from build123d import *

# Parameters (mm, degrees)
SALIENTE_EXTRUIR1_DEPTH = 0.8
SALIENTE_EXTRUIR2_DEPTH = 8
CROQUIS3_R              = 2.25
CORTAR_EXTRUIR1_DEPTH   = 0.8


with BuildPart() as part:
    # Croquis1 → Saliente-Extruir1 (new body)
    with BuildSketch(Plane.XY):
        with BuildLine():
            Line((-68.221491284, 9.846072283), (-68.221491284, 13.429873796))
            Line((-68.221491284, 13.429873796), (-62.221491284, 13.429873796))
            Line((-62.221491284, 13.429873796), (-62.221491284, 9.846072283))
            ThreePointArc((-62.221491284, 9.846072283), (-59.564637034, 8.086728046), (-57.805292797, 5.429873796))
            Line((-57.805292797, 5.429873796), (-54.221491284, 5.429873796))
            Line((-54.221491284, 5.429873796), (-54.221491284, -0.570126204))
            Line((-54.221491284, -0.570126204), (-57.805292797, -0.570126204))
            ThreePointArc((-57.805292797, -0.570126204), (-59.564637034, -3.226980453), (-62.221491284, -4.986324691))
            Line((-62.221491284, -4.986324691), (-62.221491284, -8.570126204))
            Line((-62.221491284, -8.570126204), (-68.221491284, -8.570126204))
            Line((-68.221491284, -8.570126204), (-68.221491284, -4.986324691))
            ThreePointArc((-68.221491284, -4.986324691), (-70.878345533, -3.226980453), (-72.637689771, -0.570126204))
            Line((-72.637689771, -0.570126204), (-76.221491284, -0.570126204))
            Line((-76.221491284, -0.570126204), (-76.221491284, 5.429873796))
            Line((-76.221491284, 5.429873796), (-72.637689771, 5.429873796))
            ThreePointArc((-72.637689771, 5.429873796), (-70.878345533, 8.086728046), (-68.221491284, 9.846072283))
        make_face()
    extrude(amount=SALIENTE_EXTRUIR1_DEPTH)

    # Croquis2 → Saliente-Extruir2 (add)
    with BuildSketch(Plane.XY.offset(0.8)):
        with BuildLine():
            Line((-72.637689771, -0.570126204), (-76.221491284, -0.570126204))
            Line((-76.221491284, -0.570126204), (-76.221491284, 1.929873796))
            Line((-76.221491284, 1.929873796), (-75.421491284, 1.929873796))
            Line((-75.421491284, 1.929873796), (-75.421491284, 0.229873796))
            Line((-75.421491284, 0.229873796), (-72.221491284, 0.229873796))
            ThreePointArc((-72.221491284, 0.229873796), (-70.409939992, -2.758574912), (-67.421491284, -4.570126204))
            Line((-67.421491284, -4.570126204), (-67.421491284, -7.770126204))
            Line((-67.421491284, -7.770126204), (-65.721491284, -7.770126204))
            Line((-65.721491284, -7.770126204), (-65.721491284, -8.570126204))
            Line((-65.721491284, -8.570126204), (-68.221491284, -8.570126204))
            Line((-68.221491284, -8.570126204), (-68.221491284, -4.986324691))
            ThreePointArc((-68.221491284, -4.986324691), (-70.878345533, -3.226980453), (-72.637689771, -0.570126204))
        make_face()
        with BuildLine():
            Line((-76.221491284, 5.429873796), (-72.637689771, 5.429873796))
            ThreePointArc((-72.637689771, 5.429873796), (-70.878345533, 8.086728046), (-68.221491284, 9.846072283))
            Line((-68.221491284, 9.846072283), (-68.221491284, 13.429873796))
            Line((-68.221491284, 13.429873796), (-65.721491284, 13.429873796))
            Line((-65.721491284, 13.429873796), (-65.721491284, 12.629873796))
            Line((-65.721491284, 12.629873796), (-67.421491284, 12.629873796))
            Line((-67.421491284, 12.629873796), (-67.421491284, 9.429873796))
            ThreePointArc((-67.421491284, 9.429873796), (-70.409939992, 7.618322504), (-72.221491284, 4.629873796))
            Line((-72.221491284, 4.629873796), (-75.421491284, 4.629873796))
            Line((-75.421491284, 4.629873796), (-75.421491284, 2.929873796))
            Line((-75.421491284, 2.929873796), (-76.221491284, 2.929873796))
            Line((-76.221491284, 2.929873796), (-76.221491284, 5.429873796))
        make_face()
        with BuildLine():
            Line((-62.221491284, 13.429873796), (-62.221491284, 9.846072283))
            ThreePointArc((-62.221491284, 9.846072283), (-59.564637034, 8.086728046), (-57.805292797, 5.429873796))
            Line((-57.805292797, 5.429873796), (-54.221491284, 5.429873796))
            Line((-54.221491284, 5.429873796), (-54.221491284, 2.929873796))
            Line((-54.221491284, 2.929873796), (-55.021491284, 2.929873796))
            Line((-55.021491284, 2.929873796), (-55.021491284, 4.629873796))
            Line((-55.021491284, 4.629873796), (-58.221491284, 4.629873796))
            ThreePointArc((-58.221491284, 4.629873796), (-60.033042575, 7.618322504), (-63.021491284, 9.429873796))
            Line((-63.021491284, 9.429873796), (-63.021491284, 12.629873796))
            Line((-63.021491284, 12.629873796), (-64.721491284, 12.629873796))
            Line((-64.721491284, 12.629873796), (-64.721491284, 13.429873796))
            Line((-64.721491284, 13.429873796), (-62.221491284, 13.429873796))
        make_face()
        with BuildLine():
            Line((-54.221491284, -0.570126204), (-57.805292797, -0.570126204))
            ThreePointArc((-57.805292797, -0.570126204), (-59.564637034, -3.226980453), (-62.221491284, -4.986324691))
            Line((-62.221491284, -4.986324691), (-62.221491284, -8.570126204))
            Line((-62.221491284, -8.570126204), (-64.721491284, -8.570126204))
            Line((-64.721491284, -8.570126204), (-64.721491284, -7.770126204))
            Line((-64.721491284, -7.770126204), (-63.021491284, -7.770126204))
            Line((-63.021491284, -7.770126204), (-63.021491284, -4.570126204))
            ThreePointArc((-63.021491284, -4.570126204), (-60.033042575, -2.758574912), (-58.221491284, 0.229873796))
            Line((-58.221491284, 0.229873796), (-55.021491284, 0.229873796))
            Line((-55.021491284, 0.229873796), (-55.021491284, 1.929873796))
            Line((-55.021491284, 1.929873796), (-54.221491284, 1.929873796))
            Line((-54.221491284, 1.929873796), (-54.221491284, -0.570126204))
        make_face()
    extrude(amount=SALIENTE_EXTRUIR2_DEPTH)

    # Croquis3 → Cortar-Extruir1 (cut)
    with BuildSketch(Plane.XY.offset(0.8)):
        with Locations((-65.221491284, 2.429873796)):
            Circle(CROQUIS3_R)
    extrude(amount=-CORTAR_EXTRUIR1_DEPTH, mode=Mode.SUBTRACT)


solid = part.part
Check sheet for the modelled part. Datum: model origin and axes. Units: mm. A direction names the side the tool comes from. Give positions to 0.01 mm unless a question says otherwise; leave off trailing zeros. Loops run counter-clockwise (first coordinate to the right, second up) from the corner with the lowest first, then second, coordinate; pieces in that order, holes last. Notation, with made-up numbers: M -29,-27.5 L -3,-27.5 A19 cw -3,-7.5 Z; hole C 79,50.5 d8. An arc over 180 degrees is marked long. Use a Markdown table: item, result. Add a question column.
Q1. Scan lines: line 1 along X through (y, z) = (11.25, 2); line 2 along X through (y, z) = (4, 2.5); line 3 along Y through (x, z) = (-66, 1). Record each from-to range of solid material in increasing order. Write a range as [from, to].
Q2. Sectioned sample at D-D, the plane z = 8. Give the number of separate pieces and of enclosed holes in the cut face, then the cut area to 3 significant figures.
Q3. Sectioned sample at A-A, the plane x = -56.5. Record the cut outline in (y, z), then the cut area to 3 significant figures.
Q4. Sectioned sample at B-B, the plane y = -5.75. Record the cut outline in (x, z), then the cut area to 3 significant figures.
Q5. Tool access check on faces 1 (the flat face through (-62.221, -7, 4)), 2 (the flat face through (-62.221, 12, 4)), 3 (the cylindrical face through (-70.91, 8.055, 4.338)), 4 (the flat face through (-74, -0.57, 4)), 5 (the flat face through (-67.421, -6, 5)). Record the directions out of +Z, -Z, +X, -X, +Y, -Y that give a thin tool (end or side, any length) a straight path to the whole face; none if there is none.
Q6. Go/stop test with flat-tipped pins: pin 1 (5 mm diameter, centred on x = -69, y = 0.5, fed in from +Z); pin 2 (0.6 mm diameter, centred on x = -75.5, z = 5.5, fed in from -Y); pin 3 (1 mm diameter, centred on y = -7, z = 4.5, fed in from -X). Record where each tip stops, or that it passes through.
Q7. Sectioned sample at C-C, the plane x = -67. Record the cut outline in (y, z), then the cut area to 3 significant figures.
Q8. Mould release check, pull along Y, two halves, no side actions. Record for faces 6 (the flat face through (-56, 5.43, 4)), 7 (the flat face through (-75.421, 1, 5)), 8 (the flat face through (-70.56, -3.3, 8.8)): pulls with the +Y half, pulls with the -Y half, needs draft (parallel to the pull), parting line crosses it, or undercut.
Verdict:
| question | item | result |
|---|---|---|
| 1 | line 1 | [-68.22, -67.42], [-63.02, -62.22] |
| 1 | line 2 | [-76.22, -75.42], [-55.02, -54.22] |
| 1 | line 3 | [-8.57, -7.77], [12.63, 13.43] |
| 2 | separate pieces | 4 |
| 2 | enclosed holes | 0 |
| 2 | area | 53.0 mm^2 |
| 3 | outline | M -0.57,0 L 5.43,0 L 5.43,8.8 L 4.63,8.8 L 4.63,0.8 L 0.23,0.8 L 0.23,8.8 L -0.57,8.8 Z |
| 3 | area | 17.6 mm^2 |
| 4 | outline | M -68.22,0 L -62.22,0 L -62.22,8.8 L -63.02,8.8 L -63.02,0.8 L -67.42,0.8 L -67.42,8.8 L -68.22,8.8 Z |
| 4 | area | 17.6 mm^2 |
| 5 | face 1 | +Z, -Z, +X, -Y |
| 5 | face 2 | +Z, -Z, +X, +Y |
| 5 | face 3 | +Z, -Z, -X, +Y |
| 5 | face 4 | +Z, -Z, -X, -Y |
| 5 | face 5 | +Z |
| 6 | pin 1 | z = 0.8 |
| 6 | pin 2 | y = -0.57 |
| 6 | pin 3 | x = -68.22 |
| 7 | outline | M -8.57,0 L 1.05,0 L 1.05,0.8 L -7.77,0.8 L -7.77,8.8 L -8.57,8.8 Z; M 3.81,0 L 13.43,0 L 13.43,8.8 L 12.63,8.8 L 12.63,0.8 L 3.81,0.8 Z |
| 7 | area | 28.2 mm^2 |
| 8 | face 6 | pulls with the +Y half |
| 8 | face 7 | undercut |
| 8 | face 8 | needs draft |
